Part print with two shaded views. Sizes in mm from the minimum x, y, z corner. A direction names the side the tool comes from. Round coordinates to 2 decimals unless told otherwise and drop trailing zeros. Order: outer loops, then holes, each group sorted by start corner. A loop starts at its lowest first (then second) coordinate and runs counter-clockwise, first axis right, second up. Notation, with made-up numbers: M 72,62 L 88,62 A23 cw 88,83 Z; hole C 28,40.5 d6. An arc over 180 degrees is marked long. Return JSON: item names as keys, results as strings. Group by question number.
Item 1: Slice it at C-C on x = 56. Write the cut outline in (y, z), then the cut area to 3 significant figures.
Item 2: Slice it at A-A on z = 17. Write the cut outline in (x, y), then the cut area to 3 significant figures.
Item 3: Probe line 1 along X through (y, z) = (5.25, 16.25); line 2 along Z through (x, y) = (48, 13); line 3 along Y through (x, z) = (45.5, 1.5). List the from-to ranges inside material, lowest first.
Item 4: Slice it at D-D on x = 8. Write the cut outline in (y, z), then the cut area to 3 significant figures.
Item 5: Slice it at B-B on y = 12.5. Write the cut outline in (x, z), then the cut area to 3 significant figures.
Item 6: Which spindle directions (+Z, -Z, +X, -X, +Y, -Y) get a long thin tool onto all of the face, cutting with end or side? Do the marked faces 1, 2 and 3. Say none if no direction does.
Item 7: Pull direction X, two halves, no side cores. Call the marked faces 4, 5 and 6: pulls with the +X half, pulls with the -X half, needs draft (parallel to the pull), parting line crosses it, or undercut.
Item 8: Pin check, flat tips, straight feed: pin 1 Ø0.9 at (x, z) = (48, 17) entering from +Y; pin 2 Ø2 at (x, y) = (35.5, 11) entering from -Z. Stop position of each tip, or through.
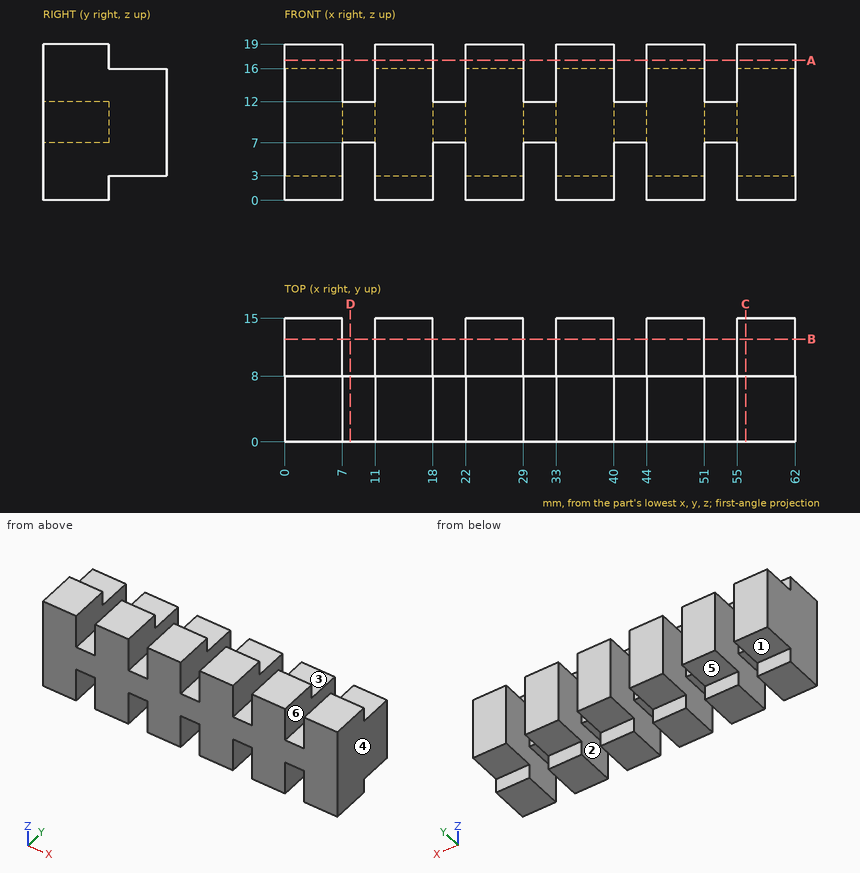
Output values:
{
 "1": {"outline": "M 0,0 L 8,0 L 8,3 L 15,3 L 15,16 L 8,16 L 8,19 L 0,19 Z", "area": "243 mm²"},
 "2": {"outline": "M 0,0 L 7,0 L 7,8 L 0,8 Z; M 11,0 L 18,0 L 18,8 L 11,8 Z; M 22,0 L 29,0 L 29,8 L 22,8 Z; M 33,0 L 40,0 L 40,8 L 33,8 Z; M 44,0 L 51,0 L 51,8 L 44,8 Z; M 55,0 L 62,0 L 62,8 L 55,8 Z", "area": "336 mm²"},
 "3": {"line 1": "0 to 7, 11 to 18, 22 to 29, 33 to 40, 44 to 51, 55 to 62", "line 2": "3 to 16", "line 3": "0 to 8"},
 "4": {"outline": "M 0,7 L 8,7 L 8,12 L 0,12 Z", "area": "40.0 mm²"},
 "5": {"outline": "M 0,3 L 7,3 L 7,16 L 0,16 Z; M 11,3 L 18,3 L 18,16 L 11,16 Z; M 22,3 L 29,3 L 29,16 L 22,16 Z; M 33,3 L 40,3 L 40,16 L 33,16 Z; M 44,3 L 51,3 L 51,16 L 44,16 Z; M 55,3 L 62,3 L 62,16 L 55,16 Z", "area": "546 mm²"},
 "6": {"face 1": "-Z, +X, -X, +Y", "face 2": "+Y", "face 3": "+Z, +X, -X, +Y"},
 "7": {"face 4": "pulls with the +X half", "face 5": "needs draft", "face 6": "undercut"},
 "8": {"pin 1": "y = 8", "pin 2": "z = 3"}
}
